For this review, take the finished solid that the model builds, in its own axes (mm). A direction names the side the tool comes from. Round coordinates to 2 decimals unless told otherwise and drop trailing zeros. Loops run counter-clockwise (first coordinate to the right, second up) from the corner with the lowest first, then second, coordinate; pieces in that order, holes last.
1. Consider section C-C on z = 4.2. State how many separate pieces and enclosed holes the cut face has, then the cut area to 3 significant figures.
2. Draft analysis for pull direction Y (two halves, no side actions). For faces 3 (the flat face through (-2, 12, 0)), 4 (the flat face through (-58.23, 158.74, 2.46)), 5 (the flat face through (50.71, 155.77, 2.46)), state which applies: released by +Y, released by -Y, zero draft, split by the parting line, or undercut.
3. Consider section A-A on y = -38. State the section outline as (x, z) points, then the cut area to 3 significant figures.
4. Consider section B-B on x = -5. State the section outline as (y, z) points.
5. To check wall thickness, follow line 1 along X through (y, z) = (148, 2.4); line 2 along X through (y, z) = (-52, 3.55); line 3 along Y through (x, z) = (-54.5, 3.7). State the ranges of each line that lie inside material, in increasing order.
6. Consider section D-D on y = 59. State the section outline as (x, z) points, then the cut area to 3 significant figures.
7. Tool access review of faces 1 (the flat face through (166.59, -28.94, 2.46)), 2 (the flat face through (-160.253, -33.967, 2.465)): name each direction out of +Z, -Z, +X, -X, +Y, -Y from which nothing blocks a thin tool from reaching the whole face with its end or side.
8. Clearance check with flat-ended pins moving along their axes: pin 1 Ø1 at (y, z) = (84, 1) entering from +X; pin 2 Ø1.5 at (x, z) = (100, 3) entering from -Y; pin 3 Ø1.8 at (x, z) = (-122.5, 3) entering from +Y; pin 4 Ø6 at (x, y) = (24, 38.5) entering from -Z. State where each tip first meets the part, or that it passes through.
from build123d import *

# Parameters (mm, degrees)
F1_DEPTH = 5
F2_R     = 5
F3_R     = 5
F4_R     = 25


# Not quite as in the source:
# - ends of sketch curves that miss each other by under 0.0002 mm in the source are joined


with BuildPart() as f1:
    # F0 (on Top) → F1 (new body)
    with BuildSketch(Plane.XY):
        with BuildLine():
            ThreePointArc((154.7685858954, -8.4666888412), (154.9421356729, -4.2349253955), (155, 0))
            ThreePointArc((155, 0), (132.0663621555, 81.1386220428), (70.0519227484, 138.2668728194))
            ThreePointArc((70.0519227484, 138.2668728194), (62.8960752724, 141.6653934994), (55.5759359282, 144.6938676852))
            ThreePointArc((55.5759359282, 144.6938676852), (53.8706420703, 143.993176318), (52.3166727987, 144.9852322827))
            Line((52.3166727987, 144.9852322827), (51.6490211362, 146.1416388839))
            ThreePointArc((51.6490211362, 146.1416388839), (46.0520817915, 148.0006951425), (40.3884712615, 149.6454856959))
            ThreePointArc((40.3884712615, 149.6454856959), (2.3057e-06, 155), (-40.3884668093, 149.6454868975))
            ThreePointArc((-40.3884668093, 149.6454868975), (-46.0520770675, 148.0006966124), (-51.6490161547, 146.1416406444))
            Line((-51.6490161547, 146.1416406445), (-52.3166688853, 144.9852321932))
            ThreePointArc((-52.3166688853, 144.9852321932), (-53.8706389409, 143.9931761584), (-55.5759330313, 144.6938687979))
            ThreePointArc((-55.5759330313, 144.6938687979), (-62.8960721537, 141.665394884), (-70.0519194288, 138.2668745012))
            ThreePointArc((-70.0519194288, 138.2668745012), (-134.2339375866, 77.5), (-154.7685855343, -8.4666954414))
            ThreePointArc((-154.7685855343, -8.4666954414), (-154.1338668835, -16.3631011587), (-153.0965326665, -24.2167645548))
            ThreePointArc((-153.0965326665, -24.2167645548), (-151.9167610651, -24.9023775772), (-151.4512795032, -26.1850518006))
            ThreePointArc((-151.4512795032, -26.1850518006), (-151.5194278506, -26.7026898908), (-151.7192286956, -27.1850518006))
            Line((-151.7192286956, -27.1850518006), (-152.3868814262, -28.3414602518))
            ThreePointArc((-152.3868814262, -28.3414602518), (-151.1984015779, -34.1180796687), (-149.7910266196, -39.845305172))
            ThreePointArc((-149.7910266196, -39.845305172), (-134.2339373892, -77.500000342), (-109.4025592509, -109.8001822829))
            ThreePointArc((-109.4025592509, -109.8001822829), (-105.1463222254, -113.8826190535), (-100.7378611443, -117.800183922))
            Line((-100.7378611443, -117.8001839221), (-99.4025592509, -117.8001839221))
            ThreePointArc((-99.4025592509, -117.8001839221), (-97.9883456885, -118.3859703597), (-97.4025592509, -119.8001839221))
            ThreePointArc((-97.4025592509, -119.8001839221), (-97.4322899717, -120.143751918), (-97.5205982187, -120.4771053897))
            ThreePointArc((-97.5205982187, -120.4771053897), (-91.2377891853, -125.3022977626), (-84.7166561444, -129.8001855612))
            ThreePointArc((-84.7166561444, -129.8001855612), (0, -155), (84.7166561444, -129.8001855612))
            ThreePointArc((84.7166561444, -129.8001855612), (91.2377891853, -125.3022977626), (97.5205982187, -120.4771053897))
            ThreePointArc((97.5205982187, -120.4771053897), (97.7664292231, -118.6499324137), (99.4025592509, -117.8001839221))
            Line((99.4025592509, -117.8001839221), (100.7378611443, -117.8001839221))
            ThreePointArc((100.7378611443, -117.800183922), (105.1463222254, -113.8826190535), (109.4025592509, -109.8001822829))
            ThreePointArc((109.4025592509, -109.8001822829), (134.233938542, -77.4999983451), (149.791027805, -39.8453007155))
            ThreePointArc((149.791027805, -39.8453007155), (151.1984026669, -34.1180748426), (152.3868823923, -28.3414550574))
            Line((152.3868823923, -28.3414550574), (151.719230036, -27.1850472546))
            ThreePointArc((151.719230036, -27.1850472546), (151.6370691989, -25.3432419871), (153.0965333673, -24.2167601241))
            ThreePointArc((153.0965333673, -24.2167601241), (154.1338674692, -16.3630956418), (154.7685858954, -8.4666888412))
        make_face()
        with BuildLine():
            ThreePointArc((55.5759359282, 144.6938676852), (62.8960752724, 141.6653934994), (70.0519227484, 138.2668728194))
            Line((70.0519227484, 138.2668728194), (47.7089766448, 176.9659938193))
            Line((47.7089766448, 176.9659938193), (30.3884705677, 166.9659949732))
            Line((30.3884705677, 166.9659949732), (40.3884712615, 149.6454856959))
            ThreePointArc((40.3884712615, 149.6454856959), (46.0520817915, 148.0006951425), (51.6490211362, 146.1416388839))
            Line((51.6490211362, 146.1416388839), (42.3166727987, 162.3057403584))
            ThreePointArc((42.3166727987, 162.3057403584), (43.0487236063, 165.037791166), (45.7807744138, 164.3057403584))
            Line((45.7807744138, 164.3057403584), (55.7807744138, 146.9852322827))
            ThreePointArc((55.7807744138, 146.9852322827), (55.9805752588, 146.5028703729), (56.0487236063, 145.9852322827))
            ThreePointArc((56.0487236063, 145.9852322827), (55.9268110169, 145.2976367053), (55.5759359282, 144.6938676852))
        make_face()
        with BuildLine():
            Line((177.1115338821, -47.1658099451), (154.7685858954, -8.4666888412))
            ThreePointArc((154.7685858954, -8.4666888412), (154.1338674692, -16.3630956418), (153.0965333673, -24.2167601241))
            ThreePointArc((153.0965333673, -24.2167601241), (154.2930861111, -24.3708356099), (155.1833316512, -25.1850472546))
            Line((155.1833316512, -25.1850472546), (165.1833316512, -42.5055553303))
            ThreePointArc((165.1833316512, -42.5055553303), (165.3831324962, -42.9879172401), (165.4512808436, -43.5055553303))
            ThreePointArc((165.4512808436, -43.5055553303), (163.9689189338, -45.4374069829), (161.719230036, -44.5055553303))
            Line((161.719230036, -44.5055553303), (152.3868823923, -28.3414550574))
            ThreePointArc((152.3868823923, -28.3414550574), (151.1984026669, -34.1180748426), (149.791027805, -39.8453007155))
            Line((149.791027805, -39.8453007155), (159.791027805, -57.1658087912))
            Line((159.791027805, -57.1658087912), (177.1115338821, -47.1658099451))
        make_face()
        with BuildLine():
            ThreePointArc((-51.6490161547, 146.1416406444), (-46.0520770675, 148.0006966124), (-40.3884668093, 149.6454868975))
            Line((-40.3884668093, 149.6454868975), (-30.3884668093, 166.9659949732))
            Line((-30.3884668093, 166.9659949732), (-47.7089725764, 176.9659936403))
            Line((-47.7089725764, 176.9659936403), (-70.0519194288, 138.2668745012))
            ThreePointArc((-70.0519194288, 138.2668745012), (-62.8960721537, 141.665394884), (-55.5759330313, 144.6938687979))
            ThreePointArc((-55.5759330313, 144.6938687979), (-56.0407757277, 145.8071514412), (-55.7807705004, 146.9852321932))
            Line((-55.7807705004, 146.9852321932), (-45.7807705004, 164.3057402689))
            ThreePointArc((-45.7807705004, 164.3057402689), (-43.5310816027, 165.2375919215), (-42.0487196929, 163.3057402689))
            ThreePointArc((-42.0487196929, 163.3057402689), (-42.1168680403, 162.7881021787), (-42.3166688853, 162.3057402689))
            Line((-42.3166688853, 162.3057402689), (-51.6490161547, 146.1416406445))
        make_face()
        with BuildLine():
            Line((129.4025592509, -109.8001822829), (109.4025592509, -109.8001822829))
            ThreePointArc((109.4025592509, -109.8001822829), (105.1463222254, -113.8826190535), (100.7378611443, -117.800183922))
            Line((100.7378611443, -117.800183922), (119.4025592509, -117.8001839221))
            ThreePointArc((119.4025592509, -117.8001839221), (120.8167728132, -118.3859703597), (121.4025592509, -119.8001839221))
            ThreePointArc((121.4025592509, -119.8001839221), (120.8167728132, -121.2143974844), (119.4025592509, -121.8001839221))
            Line((119.4025592509, -121.8001839221), (99.4025592509, -121.8001842499))
            ThreePointArc((99.4025592509, -121.8001842499), (98.2523077425, -121.4363139498), (97.5205982187, -120.4771053897))
            ThreePointArc((97.5205982187, -120.4771053897), (91.2377891853, -125.3022977626), (84.7166561444, -129.8001855612))
            Line((84.7166561444, -129.8001855612), (129.4025592509, -129.8001855612))
            Line((129.4025592509, -129.8001855612), (129.4025592509, -109.8001822829))
        make_face()
        with BuildLine():
            ThreePointArc((-153.0965326665, -24.2167645548), (-154.1338668835, -16.3631011587), (-154.7685855343, -8.4666954414))
            Line((-154.7685855343, -8.4666954414), (-177.1115323867, -47.1658145805))
            Line((-177.1115323867, -47.1658145805), (-159.7910266196, -57.1658132477))
            Line((-159.7910266196, -57.1658132477), (-149.7910266196, -39.845305172))
            ThreePointArc((-149.7910266196, -39.845305172), (-151.1984015779, -34.1180796687), (-152.3868814262, -28.3414602518))
            Line((-152.3868814262, -28.3414602518), (-161.7192286956, -44.5055598762))
            ThreePointArc((-161.7192286956, -44.5055598762), (-164.4512795032, -45.2376106838), (-165.1833303107, -42.5055598762))
            Line((-165.1833303107, -42.5055598762), (-155.1833303107, -25.1850518006))
            ThreePointArc((-155.1833303107, -25.1850518006), (-154.2930850654, -24.3708402927), (-153.0965326665, -24.2167645548))
        make_face()
        with BuildLine():
            Line((-129.4025592509, -129.8001855612), (-84.7166561444, -129.8001855612))
            ThreePointArc((-84.7166561444, -129.8001855612), (-91.2377891853, -125.3022977626), (-97.5205982187, -120.4771053897))
            ThreePointArc((-97.5205982187, -120.4771053897), (-98.2523077425, -121.4363139498), (-99.4025592509, -121.8001839221))
            Line((-99.4025592509, -121.8001839221), (-119.4025592509, -121.8001839221))
            ThreePointArc((-119.4025592509, -121.8001839221), (-121.4025592509, -119.8001839221), (-119.4025592509, -117.8001839221))
            Line((-119.4025592509, -117.8001839221), (-100.7378611443, -117.8001839221))
            ThreePointArc((-100.7378611443, -117.800183922), (-105.1463222254, -113.8826190535), (-109.4025592509, -109.8001822829))
            Line((-109.4025592509, -109.8001822829), (-129.4025592509, -109.8001822829))
            Line((-129.4025592509, -109.8001822829), (-129.4025592509, -129.8001855612))
        make_face()
    extrude(amount=F1_DEPTH)

    # F2
    f2_edges = [f1.edges().sort_by_distance(p)[0] for p in [
        (-47.708973, 176.965994, 2.5),
        (-30.388467, 166.965995, 2.5),
        (30.388471, 166.965995, 2.5),
        (47.708977, 176.965994, 2.5),
        (177.111534, -47.16581, 2.5),
        (-177.111532, -47.165815, 2.5),
        (-129.402559, -109.800182, 2.5),
        (129.402559, -109.800182, 2.5),
        (159.791028, -57.165809, 2.5),
        (129.402559, -129.800186, 2.5),
        (-129.402559, -129.800186, 2.5),
        (-159.791027, -57.165813, 2.5),
    ]]
    fillet(f2_edges, radius=F2_R)

    # F3
    f3_edges = [f1.edges().sort_by_distance(p)[0] for p in [
        (-149.791027, -39.845305, 2.5),
        (149.791028, -39.845301, 2.5),
        (40.388471, 149.645486, 2.5),
        (-40.388467, 149.645487, 2.5),
        (-109.402559, -109.800182, 2.5),
        (109.402559, -109.800182, 2.5),
    ]]
    fillet(f3_edges, radius=F3_R)

    # F4
    f4_edges = [f1.edges().sort_by_distance(p)[0] for p in [
        (-70.051919, 138.266875, 2.5),
        (-154.768586, -8.466695, 2.5),
        (70.051923, 138.266873, 2.5),
        (154.768586, -8.466689, 2.5),
        (-84.716656, -129.800186, 2.5),
        (84.716656, -129.800186, 2.5),
    ]]
    fillet(f4_edges, radius=F4_R)


solid = f1.part
Resolved:
1. separate pieces: 1
1. enclosed holes: 6
1. area: 78,800 mm2
2. face 3: zero draft
2. face 4: released by +Y
2. face 5: undercut
3. outline: (-171.82, 0) - (-162.58, 0) - (-162.58, 5) - (-171.82, 5) - close; (-157.96, 0) - (157.96, 0) - (157.96, 5) - (-157.96, 5) - close; (162.58, 0) - (171.82, 0) - (171.82, 5) - (162.58, 5) - close
3. area: 1,670 mm2
4. outline: (-154.92, 0) - (154.92, 0) - (154.92, 5) - (-154.92, 5) - close
5. line 1: x = -64.43 to -55.19, -50.58 to 50.58, 55.19 to 64.43
5. line 2: x = -168.74 to -156.81, -146.02 to 146.02, 156.81 to 168.74
5. line 3: y = -145.1 to 144.04, 149.2 to 165.2
6. outline: (-143.33, 0) - (143.33, 0) - (143.33, 5) - (-143.33, 5) - close
6. area: 1,430 mm2
7. face 1: +Z, -Z, +X, +Y
7. face 2: +Z, -Z
8. pin 1: stops at x = 130.59
8. pin 2: stops at y = -129.8
8. pin 3: stops at y = 96.12
8. pin 4: stops at z = 0
